Here's how the part is built. I have some questions about the finished solid (model axes, mm). Coordinates: 2 decimals unless noted, no trailing zeros. Write each loop counter-clockwise with the first axis right and the second up, starting at its lowest first coordinate (ties: lowest second). Pieces come first, ordered by that corner, then holes.
Item 1: I'm going to push a flat-ended pin straight in: P1, Ø1.5, axis at y = 40, z = 2, coming from the +X side. Where does the tip first touch, or does it pass through?
Item 2: I want a section at A-A (z = 2.05). Count the separate pieces of the cut face and the enclosed holes in it, and give its area (3 significant figures).
Item 3: I want a section at D-D (x = 122). Please give me the cut outline in (y, z).
Item 4: I want a section at C-C (y = 18). Please give me the cut outline in (x, z), and give its area (3 significant figures).
Item 5: Please list where these lines run through material, in increasing order: line 1 (Y direction, x = 122, z = 0.7); line 2 (Y direction, x = 17.5, z = 2.2); line 3 (Y direction, x = 46, z = 1.05).
Item 6: I want a section at B-B (x = 67.5). Please give me the cut outline in (y, z).
from build123d import *

# Parameters (mm, degrees)
EXTRUDE_1_DEPTH     = 3
SKETCH_2_W          = 14
SKETCH_2_H          = 9
CUT_EXTRUDE_1_DEPTH = 167.460205455
SKETCH_3_W          = 67
SKETCH_3_H          = 52
CUT_EXTRUDE_2_DEPTH = 167.460205455
SKETCH_4_R          = 6
CUT_EXTRUDE_3_DEPTH = 167.460205455


with BuildPart() as part:
    # Эскиз1 → Бобышка-Вытянуть1 (new body)
    with BuildSketch(Plane.XY):
        Polygon((0, 0), (40, 0), (40, 3), (100, 3), (100, 0), (140, 0), (140, 25), (137, 25), (137, 65), (140, 65), (140, 90), (100, 90), (100, 87), (40, 87), (40, 90), (0, 90), (0, 65), (3, 65), (3, 25), (0, 25), align=None)
    extrude(amount=EXTRUDE_1_DEPTH)

    # Эскиз2 → Вырез-Вытянуть1 (cut, through all)
    with BuildSketch(Plane.XY.offset(3)):
        with Locations((22, 8.5)):
            Rectangle(SKETCH_2_W, SKETCH_2_H)
    extrude(amount=-CUT_EXTRUDE_1_DEPTH, mode=Mode.SUBTRACT)

    # Эскиз3 → Вырез-Вытянуть2 (cut, through all)
    with BuildSketch(Plane.XY.offset(3)):
        with Locations((48.5, 47)):
            Rectangle(SKETCH_3_W, SKETCH_3_H)
    extrude(amount=-CUT_EXTRUDE_2_DEPTH, mode=Mode.SUBTRACT)

    # Эскиз4 → Вырез-Вытянуть3 (cut, through all)
    with BuildSketch(Plane.XY.offset(3)):
        with Locations((122, 72)):
            Circle(SKETCH_4_R)
        with Locations((122, 54)):
            Circle(SKETCH_4_R)
        with Locations((122, 36)):
            Circle(SKETCH_4_R)
        with Locations((122, 18)):
            Circle(SKETCH_4_R)
    extrude(amount=-CUT_EXTRUDE_3_DEPTH, mode=Mode.SUBTRACT)


solid = part.part
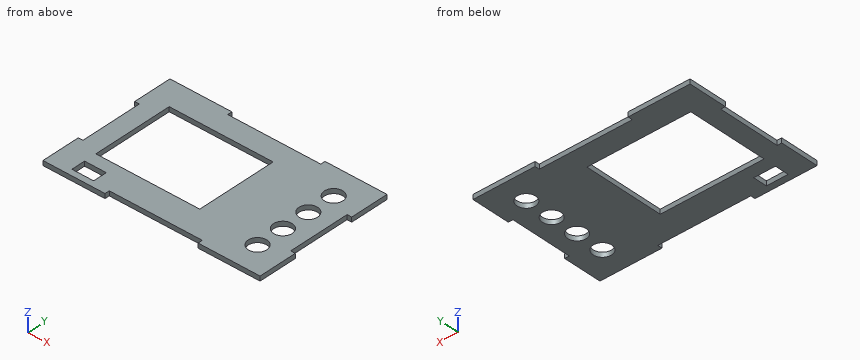
Answer:
1. P1: stops at x = 137
2. separate pieces: 1
2. enclosed holes: 6
2. area: 7,940 mm2
3. outline: (0, 0) - (12, 0) - (12, 3) - (0, 3) - close; (24, 0) - (30, 0) - (30, 3) - (24, 3) - close; (42, 0) - (48, 0) - (48, 3) - (42, 3) - close; (60, 0) - (66, 0) - (66, 3) - (60, 3) - close; (78, 0) - (90, 0) - (90, 3) - (78, 3) - close
4. outline: (0, 0) - (116, 0) - (116, 3) - (0, 3) - close; (128, 0) - (140, 0) - (140, 3) - (128, 3) - close
4. area: 384 mm2
5. line 1: y = 0 to 12, 24 to 30, 42 to 48, 60 to 66, 78 to 90
5. line 2: y = 0 to 4, 13 to 21, 73 to 90
5. line 3: y = 3 to 21, 73 to 87
6. outline: (3, 0) - (21, 0) - (21, 3) - (3, 3) - close; (73, 0) - (87, 0) - (87, 3) - (73, 3) - close
